Autodesk Inventor part; units mm, degrees
ref_plane "YZ Plane" through (0, 0, 0) normal (1, 0, 0) x (0, 1, 0)
ref_plane "XZ Plane" through (0, 0, 0) normal (0, 1, 0) x (-1, 0, 0)
ref_plane "XY Plane" through (0, 0, 0) normal (0, 0, 1) x (1, 0, 0)
sketch "Sketch1" plane through (0, 0, 0) normal (0, 0, 1) x (1, 0, 0)
  line L0 (-35.56, 0) -> (35.56, 0) construction
  line L1 (0, -35.56) -> (0, 35.56) construction
  line L2 (-25.4, 25.4) -> (25.4, 25.4)
  line L3 (25.4, 25.4) -> (25.4, -25.4)
  line L4 (25.4, -25.4) -> (-25.4, -25.4)
  line L5 (-25.4, -25.4) -> (-25.4, 25.4)
  line L6 (-22.225, 22.225) -> (22.225, 22.225)
  line L7 (22.225, 22.225) -> (22.225, -22.225)
  line L8 (22.225, -22.225) -> (-22.225, -22.225)
  line L9 (-22.225, -22.225) -> (-22.225, 22.225)
  point P0 (0, 0)
  point P1 (-25.4, 0)
  point P2 (0, 25.4)
  point P3 (-22.225, 0)
  point P4 (0, 22.225)
  dimension "d0" = 50.8
  dimension "d1" = 3.175
  dimension "d11" = 50.8
  dimension "d12" = 3.175
extrude "Extrusion1" add sketch "Sketch1" along normal mid plane 101.6
sketch "Sketch6" plane through (25.4, -25.4, 50.8) normal (1, 0, 0) x (0, 0, -1)
  circle A0 centre (50.8, 25.4) radius 14.2875
  dimension "d23" = 28.575
extrude "Extrusion7" cut sketch "Sketch6" against normal through all
sketch "Sketch7" plane through (-22.225, -22.225, -50.8) normal (1, 0, 0) x (0, 0, -1)
  circle A0 centre (-14.8971, 6.35) radius 2.667
  circle A1 centre (-86.7029, 6.35) radius 2.667
  circle A2 centre (-14.8971, 38.1) radius 2.667
  circle A3 centre (-86.7029, 38.1) radius 2.667
  point P0 (-50.8, 22.225)
extrude "Extrusion8" cut sketch "Sketch7" against normal up to next
sketch "Sketch8" plane through (25.4, -25.4, 50.8) normal (1, 0, 0) x (0, 0, -1)
  circle A0 centre (50.8, 25.4) radius 15.875 construction
  line L0 (121.92, 25.4) -> (-20.32, 25.4) construction
  circle A1 centre (69.85, 25.4) radius 3.175 construction
  line L1 (50.8, 9.525) -> (50.8, 41.275) construction
  circle A2 centre (69.85, 25.4) radius 5.5499 construction
  circle A3 centre (69.85, 25.4) radius 2.667
  circle A4 centre (31.75, 25.4) radius 2.667
  point P0 (50.8, 25.4)
  dimension "d28" = 6.35
  dimension "d29" = 11.0998
  dimension "d30" = 5.334
extrude "Extrusion9" cut sketch "Sketch8" against normal through all
equation "\"d12\" = d1"
properties part number "Arm 4 inch" material "Aluminum 6061"
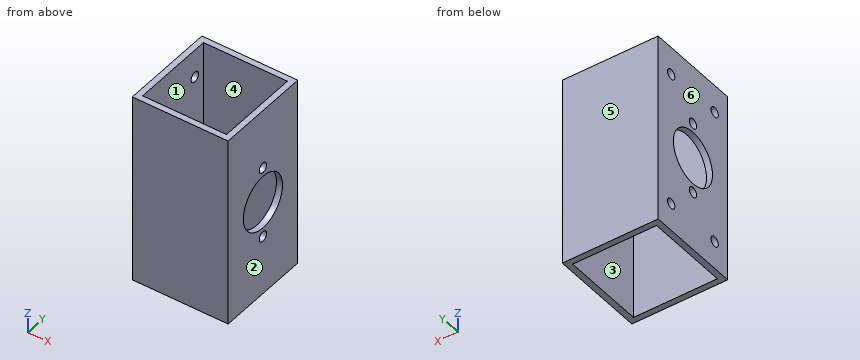
CAD build for the part. Positions are in the model's coordinates, mm. Face numbers are marked on the shaded views. A direction names the side the tool comes from. Round coordinates to 2 decimals unless told otherwise and drop trailing zeros. Write each loop counter-clockwise with the first axis right and the second up, starting at its lowest first coordinate (ties: lowest second). Pieces come first, ordered by that corner, then holes.
(1) Probe line 1 along Y through (x, z) = (-21, -44) (3 decimals); line 2 along Y through (x, z) = (-23, -19). List the from-to ranges inside material, lowest first.
(2) 3-axis set-ups, long thin cutter, end or side, ignore diameter. For the marked faces 1 and 2: which of +Z, -Z, +X, -X, +Y, -Y reach the whole face in a straight line?
(3) Slice it at D-D, the plane y = 9.5. Write the cut outline in (x, z) (3 decimals), and give its area (3 significant figures).
(4) Slice it at A-A, the plane x = -13. Write the cut outline in (y, z) (3 decimals), and give its area (3 significant figures).
(5) Mould opens along X. For the marked faces 3, 4, 5 and 6 say: pulls with the +X half, pulls with the -X half, needs draft (parallel to the pull), parting line crosses it, or undercut.
(6) Slice it at B-B, the plane y = 0. Count the separate pieces of the cut face and the enclosed holes in it, and give its area (3 significant figures).
(7) Slice it at C-C, the plane z = -19.05. Write the cut outline in (x, y) (3 decimals).
From the geometry:
1. line 1: y = -25.4 to -22.225, 22.225 to 25.4
1. line 2: y = -25.4 to -2.67, 2.67 to 25.4
2. face 1: +Z, -Z
2. face 2: +Z, -Z, +X, +Y, -Y
3. outline: (-25.4, -50.8) - (-22.225, -50.8) - (-22.225, -10.672) - (-25.4, -10.672) - close; (-25.4, 10.672) - (-22.225, 10.672) - (-22.225, 50.8) - (-25.4, 50.8) - close; (22.225, -50.8) - (25.4, -50.8) - (25.4, -10.672) - (22.225, -10.672) - close; (22.225, 10.672) - (25.4, 10.672) - (25.4, 50.8) - (22.225, 50.8) - close
3. area: 510 mm2
4. outline: (-25.4, -50.8) - (-22.225, -50.8) - (-22.225, 50.8) - (-25.4, 50.8) - close; (22.225, -50.8) - (25.4, -50.8) - (25.4, 50.8) - (22.225, 50.8) - close
4. area: 645 mm2
5. face 3: undercut
5. face 4: undercut
5. face 5: needs draft
5. face 6: pulls with the -X half
6. separate pieces: 8
6. enclosed holes: 0
6. area: 396 mm2
7. outline: (-25.4, -25.4) - (25.4, -25.4) - (25.4, -2.667) - (22.225, -2.667) - (22.225, -22.225) - (-22.225, -22.225) - (-22.225, -2.667) - (-25.4, -2.667) - close; (-25.4, 2.667) - (-22.225, 2.667) - (-22.225, 22.225) - (22.225, 22.225) - (22.225, 2.667) - (25.4, 2.667) - (25.4, 25.4) - (-25.4, 25.4) - close
